```python
from build123d import *

# Parameters (mm, degrees)
SKETCH1_W           = 106
SKETCH1_H           = 60
BOSS_EXTRUDE1_DEPTH = 10
SKETCH2_W           = 10
SKETCH2_H           = 60
BOSS_EXTRUDE2_DEPTH = 55
SKETCH3_W           = 60
SKETCH3_H           = 15
BOSS_EXTRUDE3_DEPTH = 20
SKETCH4_W           = 30
SKETCH4_H           = 15
BOSS_EXTRUDE4_DEPTH = 20
SKETCH5_R           = 4.5
CUT_EXTRUDE1_DEPTH  = 66
SKETCH6_R           = 6.5
CUT_EXTRUDE2_DEPTH  = 6.6
SKETCH7_R           = 3.3
CUT_EXTRUDE3_DEPTH  = 9.4
CUT_EXTRUDE4_DEPTH  = 66


with BuildPart() as part:
    # Sketch1 → Boss-Extrude1 (new body)
    with BuildSketch(Plane(origin=(0, 0, 0), x_dir=(1, 0, 0), z_dir=(0, 1, 0))):
        Rectangle(SKETCH1_W, SKETCH1_H)
    extrude(amount=BOSS_EXTRUDE1_DEPTH)

    # Sketch2 → Boss-Extrude2 (add)
    with BuildSketch(Plane.XZ):
        with Locations((-48, 0)):
            Rectangle(SKETCH2_W, SKETCH2_H)
        with Locations((48, 0)):
            Rectangle(SKETCH2_W, SKETCH2_H)
    extrude(amount=BOSS_EXTRUDE2_DEPTH)

    # Sketch3 → Boss-Extrude3 (add)
    with BuildSketch(Plane(origin=(53, 0, 0), x_dir=(0, 0, -1), z_dir=(1, 0, 0))):
        with Locations((0, -47.5)):
            Rectangle(SKETCH3_W, SKETCH3_H)
    extrude(amount=BOSS_EXTRUDE3_DEPTH)

    # Sketch4 → Boss-Extrude4 (add)
    with BuildSketch(Plane.ZY.offset(53)):
        with Locations((-15, -47.5)):
            Rectangle(SKETCH4_W, SKETCH4_H)
    extrude(amount=BOSS_EXTRUDE4_DEPTH)

    # Sketch5 → Cut-Extrude1 (cut, through all)
    with BuildSketch(Plane(origin=(0, 10, 0), x_dir=(1, 0, 0), z_dir=(0, 1, 0))):
        with Locations((-32, 21)):
            Circle(SKETCH5_R)
        with Locations((32, 21)):
            Circle(SKETCH5_R)
        with Locations((32, -21)):
            Circle(SKETCH5_R)
        with Locations((-32, -21)):
            Circle(SKETCH5_R)
    extrude(amount=-CUT_EXTRUDE1_DEPTH, mode=Mode.SUBTRACT)

    # Sketch6 → Cut-Extrude2 (cut)
    with BuildSketch(Plane(origin=(0, -40, 0), x_dir=(1, 0, 0), z_dir=(0, 1, 0))):
        with Locations((63, 20)):
            Circle(SKETCH6_R)
        with Locations((63, -20)):
            Circle(SKETCH6_R)
        with Locations((-63, 20)):
            Circle(SKETCH6_R)
    extrude(amount=-CUT_EXTRUDE2_DEPTH, mode=Mode.SUBTRACT)

    # Sketch7 → Cut-Extrude3 (cut, through all)
    with BuildSketch(Plane(origin=(0, -46.6, 0), x_dir=(1, 0, 0), z_dir=(0, 1, 0))):
        with Locations((-63, 20)):
            Circle(SKETCH7_R)
        with Locations((63, -20)):
            Circle(SKETCH7_R)
        with Locations((63, 20)):
            Circle(SKETCH7_R)
    extrude(amount=-CUT_EXTRUDE3_DEPTH, mode=Mode.SUBTRACT)

    # Sketch8 → Cut-Extrude4 (cut, through all)
    with BuildSketch(Plane(origin=(0, 10, 0), x_dir=(1, 0, 0), z_dir=(0, 1, 0))):
        Polygon((-38.239, -30), (-53, -3.370451084), (-53, -30), align=None)
    extrude(amount=-CUT_EXTRUDE4_DEPTH, mode=Mode.SUBTRACT)


solid = part.part
```
Here's how the part is built. I have some questions about the finished solid (model axes, mm). A direction names the side the tool comes from. Give positions to 0.01 mm unless a question says otherwise; leave off trailing zeros. Write each loop counter-clockwise with the first axis right and the second up, starting at its lowest first coordinate (ties: lowest second). Pieces come first, ordered by that corner, then holes. Notation, with made-up numbers: (-38, -25.5) -> (-27, -25.5) arc R25 ccw to (-27, -4.5) -> close; hole circle Ø1 at (81.5, 25.5). An arc over 180 degrees is marked (long way). Write each question's results on one line, items separated by ' | '.
Item 1: We'd pull the mould along X, two halves only. Please class faces 4 (the face through (6, 1, -30)), 5 (the face through (73, -47, 0)), 6 (the face through (60.381, -50.741, 22.008)): pulls with the +X half, pulls with the -X half, needs draft (parallel to the pull), parting line crosses it, or undercut.
Output:
face 4: needs draft | face 5: pulls with the +X half | face 6: undercut
Item 2: Suppose I cut it at A-A on y = -28. Write out the boundary of the cut face in (x, z), plus the area to 3 significant figures.
Output:
outline: (-53, -30) -> (-43, -30) -> (-43, 21.41) -> (-53, 3.37) -> close; (43, -30) -> (53, -30) -> (53, 30) -> (43, 30) -> close | area: 1,020 mm^2
Item 3: Suppose I cut it at B-B on x = 63. Write out the boundary of the cut face in (y, z).
Output:
outline: (-55, -30) -> (-40, -30) -> (-40, -26.5) -> (-46.6, -26.5) -> (-46.6, -23.3) -> (-55, -23.3) -> close; (-55, -16.7) -> (-46.6, -16.7) -> (-46.6, -13.5) -> (-40, -13.5) -> (-40, 13.5) -> (-46.6, 13.5) -> (-46.6, 16.7) -> (-55, 16.7) -> close; (-55, 23.3) -> (-46.6, 23.3) -> (-46.6, 26.5) -> (-40, 26.5) -> (-40, 30) -> (-55, 30) -> close
Item 4: Suppose I cut it at D-D on z = 6. Write out the boundary of the cut face in (x, y), plus the area to 3 significant figures.
Output:
outline: (-51.54, -55) -> (-43, -55) -> (-43, 0) -> (43, 0) -> (43, -55) -> (73, -55) -> (73, -40) -> (53, -40) -> (53, 10) -> (-51.54, 10) -> close | area: 2,370 mm^2
Item 5: For pin 1 Ø6 at (x, z) = (63, -20) entering from -Y; pin 2 Ø10.5 at (x, z) = (63, 20) entering from +Y; pin 3 Ø4.5 at (x, y) = (-61, -44.5) entering from +Z; pin 4 Ø16 at (x, z) = (64.5, -3) entering from +Y, each with a flat end and sliding along its axis, tell me the tip position at first contact or that it passes through.
Output:
pin 1: passes through | pin 2: stops at y = -46.6 | pin 3: stops at z = 0 | pin 4: stops at y = -40
Item 6: Suppose I cut it at C-C on x = -63. Write out the boundary of the cut face in (y, z).
Output:
outline: (-55, -30) -> (-40, -30) -> (-40, -26.5) -> (-46.6, -26.5) -> (-46.6, -23.3) -> (-55, -23.3) -> close; (-55, -16.7) -> (-46.6, -16.7) -> (-46.6, -13.5) -> (-40, -13.5) -> (-40, 0) -> (-55, 0) -> close
Item 7: On a 3-axis mill with a long thin cutter (end or side, diameter ignored), from which of +Z, -Z, +X, -X, +Y, -Y can I reach the whole of each face in a straight line? I mean faces 1 (the face through (-43, -27, -5)), 2 (the face through (69.2, -43.25, 18.05)), 3 (the face through (-63, -40, -12)). Say none if no direction works.
Output:
face 1: +Z, -Z, -Y | face 2: +Y | face 3: +Z, -Z, -X, +Y
Item 8: If I drill on L1, parallel to Z at x = -32, y = 6; L2, parallel to Z at x = 63, y = -48; L3, parallel to X at y = 3.5, z = -21, over which ranges is the centre line in solid material (lowest first)?
Output:
L1: z = -30 to -25.5, -16.5 to 16.5, 25.5 to 30 | L2: z = -30 to -23.3, -16.7 to 16.7, 23.3 to 30 | L3: x = -53 to -36.5, -27.5 to 27.5, 36.5 to 53
